The model under review builds one solid part; all positions refer to its coordinate system, in mm. Face numbers are marked on the shaded views. A direction names the side the tool comes from. Round coordinates to 2 decimals unless told otherwise and drop trailing zeros. Order: outer loops, then holes, each group sorted by start corner. A loop starts at its lowest first (then second) coordinate and runs counter-clockwise, first axis right, second up. Notation, with made-up numbers: (1, 48.5) - (52, 48.5) arc R33 cw to (52, 84.5) - close; hole circle Ø5 at (85, 57.5). An arc over 180 degrees is marked (long way). One line per question, with ' | ' between items. Start each with the question number.
Item 1: Tool access review of the marked faces 1 and 2: name each direction out of +Z, -Z, +X, -X, +Y, -Y from which nothing blocks a thin tool from reaching the whole face with its end or side.
Item 2: Add section B-B on x = 0. State the section outline as (y, z) points, and give its area (3 significant figures).
Item 3: Add section C-C on y = 6. State the section outline as (x, z) points.
Item 4: For L1, parallel to Z at x = 0.95, y = 7.75; L2, parallel to X at y = 2.5, z = -1.1; L3, parallel to Y at x = -1, z = 1.75, list the stretches that pass through material, from the lowest coordinate up. Write a range as [from, to].
Item 5: Add section A-A on z = 0. State the section outline as (x, y) points, and give its area (3 significant figures).
Item 6: Insertion check: pin 1 Ø1 at (x, y) = (1, 3.5) entering from +Z; pin 2 Ø2 at (y, z) = (4, 1) entering from -X; pin 3 Ø1 at (x, z) = (0.5, 1) entering from -Y; pin 4 Ø1 at (x, y) = (-0.5, 5) entering from +Z. Each pin has a flat end and moves straight along its axis. Give the tip position at first contact, or say it passes through.
from build123d import *

# Parameters (mm, degrees)
CUT_EXTRUDE1_DEPTH = 1


with BuildPart() as part:
    # Sketch1 → Revolve1 (revolve)
    with BuildSketch(Plane.XY, mode=Mode.PRIVATE) as revolve1_sk:
        Polygon((0, 0), (1.25, 0), (1.25, 6.5), (2.35, 7.6), (2.35, 8), (0, 8), align=None)
    revolve(revolve1_sk.sketch.rotate(Axis((0, 8, 0), (0, -1, 0)), 180), axis=Axis((0, 8, 0), (0, -1, 0)))

    # Sketch2 → Cut-Extrude1 (cut)
    with BuildSketch(Plane(origin=(0, 8, 0), x_dir=(1, 0, 0), z_dir=(0, 1, 0))):
        Polygon((0, 1), (0.15, 1), (0.15, 0.15), (1, 0.15), (1, -0.15), (0.15, -0.15), (0.15, -1), (-0.15, -1), (-0.15, -0.15), (-1, -0.15), (-1, 0.15), (-0.15, 0.15), (-0.15, 1), align=None)
    extrude(amount=-CUT_EXTRUDE1_DEPTH, mode=Mode.SUBTRACT)


solid = part.part
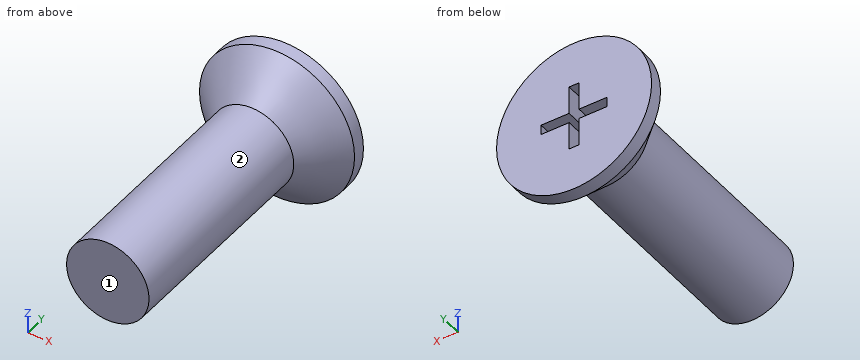
Determined:
1) face 1: +Z, -Z, +X, -X, -Y | face 2: -Y
2) outline: (0, -1.25) - (6.5, -1.25) - (7.6, -2.35) - (8, -2.35) - (8, -1) - (7, -1) - (7, 1) - (8, 1) - (8, 2.35) - (7.6, 2.35) - (6.5, 1.25) - (0, 1.25) - close | area: 20.1 mm2
3) outline: circle Ø2.5 at (0, 0)
4) L1: [-2.15, -0.15], [0.15, 2.15] | L2: [-0.59, 0.59] | L3: [7.27, 8]
5) outline: (-2.35, 7.6) - (-1.25, 6.5) - (-1.25, 0) - (1.25, 0) - (1.25, 6.5) - (2.35, 7.6) - (2.35, 8) - (1, 8) - (1, 7) - (-1, 7) - (-1, 8) - (-2.35, 8) - close | area: 20.1 mm2
6) pin 1: z = 1.15 | pin 2: x = -1.25 | pin 3: y = 0 | pin 4: z = 1.25
